Input: part model. Units: mm. Frame: model coordinates. A direction names the side the tool comes from. Give positions to 0.01 mm unless a question says otherwise; leave off trailing zeros. Write each loop counter-clockwise with the first axis right and the second up, starting at its lowest first coordinate (ties: lowest second). Pieces come first, ordered by that corner, then holes. Notation, with made-up numbers: (15.25, 54.25) - (50.25, 54.25) arc R23 ccw to (50.25, 78.25) - close; hole circle Ø1 at (-29.5, 58.5). An arc over 180 degrees is marked (long way). Use a Markdown table: item, result. Add a question column.
1. Pin query (flat end, axial travel): pin 1 (2 mm diameter, centred on y = 39, z = 25.5, fed in from -X); pin 2 (5 mm diameter, centred on x = -4, z = 7.5, fed in from +Y); pin 3 (0.9 mm diameter, centred on x = 0, y = -23, fed in from +Z). Return the tip coordinate at first contact, or that it passes through.
2. Section query A-A, the plane z = 10. Return loops of the section in (x, y).
3. Mould query, pull axis Y, two halves, no side actions, for faces 4 (the flat face through (0, -21, 3)), 5 (the flat face through (-23, -24, 26)). Classes: released by +Y, released by -Y, zero draft, split by the parting line, or undercut.
4. Material intervals for probe 1 along Z at (x, y) = (-37, 31); probe 2 along Y at (x, z) = (25.5, 32.5); probe 3 along X at (y, z) = (-1, 22), sorted ascending.
5. Set-up query: faces 1 (the cylindrical face through (-14.524, -16.314, 1.479)), 2 (the flat face through (0, 0, 34)), 3 (the cylindrical face through (27.432, -0.594, 32.521)). Return all of +Z, -Z, +X, -X, +Y, -Y with unobstructed straight access to the full face (end or side cutting, diameter ignored); none if empty.
```python
from build123d import *

# Parameters (mm, degrees)
SKETCH1_R           = 55
BOSS_EXTRUDE1_DEPTH = 26
SKETCH2_R           = 1.5
CUT_EXTRUDE1_DEPTH  = 3
SKETCH3_R           = 32.5
BOSS_EXTRUDE2_DEPTH = 8
SKETCH4_R           = 2.55
SKETCH4_R_2         = 1.55
SKETCH4_R_3         = 2.05
CUT_EXTRUDE2_DEPTH  = 3
FILLET1_R           = 2


with BuildPart() as part:
    # Sketch1 → Boss-Extrude1 (new body)
    with BuildSketch(Plane.XY):
        with Locations(Location((0, 0, 0), (0, 0, 180))):
            Circle(SKETCH1_R)
    extrude(amount=BOSS_EXTRUDE1_DEPTH)

    # Sketch2 → Cut-Extrude1 (cut)
    with BuildSketch(Plane(origin=(0, 0, 0), x_dir=(-1, 0, 0), z_dir=(0, 0, -1))):
        with Locations((0, -21)):
            Circle(SKETCH2_R)
        with Locations((-14.849242405, -14.849242405)):
            Circle(SKETCH2_R)
        with Locations((-21, 0)):
            Circle(SKETCH2_R)
        with Locations((-14.849242405, 14.849242405)):
            Circle(SKETCH2_R)
        with Locations((0, 21)):
            Circle(SKETCH2_R)
        with Locations((14.849242405, 14.849242405)):
            Circle(SKETCH2_R)
        with Locations((21, 0)):
            Circle(SKETCH2_R)
        with Locations((14.849242405, -14.849242405)):
            Circle(SKETCH2_R)
    extrude(amount=-CUT_EXTRUDE1_DEPTH, mode=Mode.SUBTRACT)

    # Sketch3 → Boss-Extrude2 (add)
    with BuildSketch(Plane.XY.offset(26)):
        Circle(SKETCH3_R)
    extrude(amount=BOSS_EXTRUDE2_DEPTH)

    # Sketch4 → Cut-Extrude2 (cut)
    with BuildSketch(Plane.XY.offset(34)):
        with Locations((-16.5, 0)):
            Circle(SKETCH4_R)
        with Locations((0, -16.5)):
            Circle(SKETCH4_R)
        with Locations((16.5, 0)):
            Circle(SKETCH4_R)
        with Locations((0, 16.5)):
            Circle(SKETCH4_R)
        with Locations((0, 26)):
            Circle(SKETCH4_R_2)
        with Locations((0, 22)):
            Circle(SKETCH4_R_2)
        with Locations((-11.66726189, -11.66726189)):
            Circle(SKETCH4_R_3)
        with Locations((11.66726189, -11.66726189)):
            Circle(SKETCH4_R_3)
        with Locations((11.66726189, 11.66726189)):
            Circle(SKETCH4_R_3)
        with Locations((-11.66726189, 11.66726189)):
            Circle(SKETCH4_R_3)
        with Locations((-22, 0)):
            Circle(SKETCH4_R_2)
        with Locations((-26, 0)):
            Circle(SKETCH4_R_2)
        with Locations((0, -22)):
            Circle(SKETCH4_R_2)
        with Locations((0, -26)):
            Circle(SKETCH4_R_2)
        with Locations((22, 0)):
            Circle(SKETCH4_R_2)
        with Locations((26, 0)):
            Circle(SKETCH4_R_2)
    extrude(amount=-CUT_EXTRUDE2_DEPTH, mode=Mode.SUBTRACT)

    # Fillet1
    fillet1_edges = [part.edges().sort_by_distance(p)[0] for p in [
        (55, 0, 0),
        (55, 0, 26),
    ]]
    fillet(fillet1_edges, radius=FILLET1_R)


solid = part.part
```
Result sheet:
| question | item | result |
|---|---|---|
| 1 | pin 1 | stops at x = -39.27 |
| 1 | pin 2 | stops at y = 54.98 |
| 1 | pin 3 | stops at z = 31 |
| 2 | outline | circle Ø110 at (0, 0) |
| 3 | face 4 | undercut |
| 3 | face 5 | zero draft |
| 4 | probe 1 | z = 0 to 26 |
| 4 | probe 2 | y = -20.15 to -1.47, 1.47 to 20.15 |
| 4 | probe 3 | x = -54.99 to 54.99 |
| 5 | face 1 | -Z |
| 5 | face 2 | +Z, +X, -X, +Y, -Y |
| 5 | face 3 | +Z |
